Read the model definition and answer for the solid it produces. Units are mm, in the model's axes. Face numbers are marked on the shaded views. A direction names the side the tool comes from. Round coordinates to 2 decimals unless told otherwise and drop trailing zeros. Write each loop counter-clockwise with the first axis right and the second up, starting at its lowest first coordinate (ties: lowest second). Pieces come first, ordered by that corner, then holes. Notation, with made-up numbers: (73, 5.25) -> (131, 5.25) arc R9 cw to (131, 15.25) -> close; hole circle Ø1 at (55, -6.75). An arc over 180 degrees is marked (long way). Return JSON: item names as keys, results as strings. Group by question number.
(1) Straight lines are drawn through the part: line 1 (X direction, y = 6.25, z = 18); line 2 (X direction, y = 6.25, z = 13); line 3 (X direction, y = 3.5, z = 0). For each, find the intervals that lie inside material, in ascending order.
(2) A cutting plane is placed at D-D on z = 0. Give the vertices of the cut face in (x, y), then the cut area to 3 significant figures.
(3) A cutting plane is placed at C-C on y = 1. Give the vertices of the cut face in (x, z).
(4) For the marked faces 4, 5, 6 and 7, determine the directions among +Z, -Z, +X, -X, +Y, -Y from which every point of the face is accessible in a straight line to the end or side of a thin tool.
(5) The mould has two halves that part along X. Classify the marked faces 1, 2 and 3: released by +X, released by -X, zero draft, split by the parting line, or undercut.
(6) A cutting plane is placed at B-B on y = 8.75. Give the vertices of the cut face in (x, z).
(7) Given pin 1 (2 mm diameter, centred on x = -0.5, z = 19.5, fed in from +Y); pin 2 (5 mm diameter, centred on x = 19.5, y = 7, fed in from -Z); pin 3 (5 mm diameter, centred on y = 7, z = 5, fed in from -X), each flat-ended and moving along its own axis, determine where each tip first touches the part or whether it passes through.
(8) A cutting plane is placed at A-A on x = 0. Give the vertices of the cut face in (y, z), then the cut area to 4 significant figures.
```python
from build123d import *

# Parameters (mm, degrees)
SKETCH1_W           = 29.5
SKETCH1_H           = 6.5
SKETCH1_R           = 1.65
SKETCH1_H_2         = 20
BOSS_EXTRUDE1_DEPTH = 5
SKETCH3_W           = 14.6
SKETCH3_H           = 13.25
SKETCH3_W_2         = 14.2
BOSS_EXTRUDE2_DEPTH = 5
SKETCH5_W           = 3
SKETCH5_H           = 13.25
BOSS_EXTRUDE4_DEPTH = 5
BOSS_EXTRUDE5_DEPTH = 2.5


with BuildPart() as part:
    # Sketch1 → Boss-Extrude1 (new body)
    # profile 1 of 2: a face of its own
    with BuildSketch(Plane(origin=(0, 0, 0), x_dir=(1, 0, 0), z_dir=(0, 1, 0))):
        Rectangle(SKETCH1_W, SKETCH1_H)
        with Locations(Location((0, 0, 0), (0, 0, 270))):
            Circle(SKETCH1_R, mode=Mode.SUBTRACT)
    # profile 2 of 2: a face of its own
    with BuildSketch(Plane(origin=(0, 0, 0), x_dir=(1, 0, 0), z_dir=(0, 1, 0))):
        with Locations((0, -13.25)):
            Rectangle(SKETCH1_W, SKETCH1_H_2)
    extrude(amount=BOSS_EXTRUDE1_DEPTH)

    # Sketch3 → Boss-Extrude2 (add)
    with BuildSketch(Plane(origin=(0, 5, 0), x_dir=(1, 0, 0), z_dir=(0, 1, 0))):
        with Locations((22.05, -16.625)):
            Rectangle(SKETCH3_W, SKETCH3_H)
        with Locations((-21.85, -16.625)):
            Rectangle(SKETCH3_W_2, SKETCH3_H)
    extrude(amount=-BOSS_EXTRUDE2_DEPTH)

    # Sketch5 → Boss-Extrude4 (add, symmetric)
    with BuildSketch(Plane(origin=(0, 5, 0), x_dir=(1, 0, 0), z_dir=(0, 1, 0))):
        with Locations((-30.45, -16.625)):
            Rectangle(SKETCH5_W, SKETCH5_H)
        with Locations((30.85, -16.625)):
            Rectangle(SKETCH5_W, SKETCH5_H)
    extrude(amount=BOSS_EXTRUDE4_DEPTH, both=True)

    # Sketch6 → Boss-Extrude5 (add)
    with BuildSketch(Plane(origin=(0, 5, 0), x_dir=(1, 0, 0), z_dir=(0, 1, 0))):
        Polygon((0, -23.25), (7, -23.25), (7, -16.25), (-7, -16.25), (-7, -23.25), align=None)
    extrude(amount=BOSS_EXTRUDE5_DEPTH)


solid = part.part
```
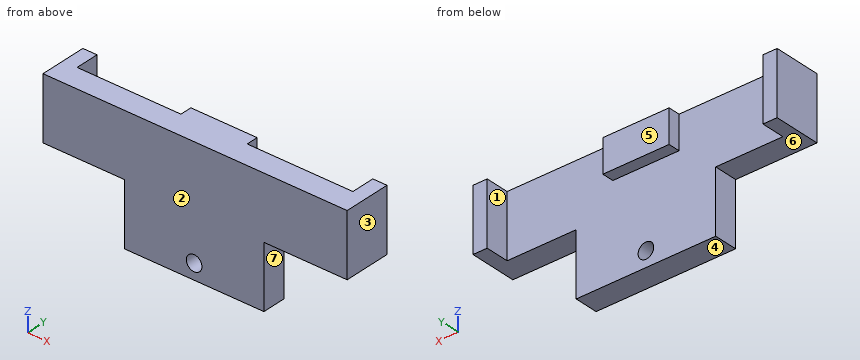
Checks:
{
 "1": {"line 1": "x = -31.95 to -28.95, -7 to 7, 29.35 to 32.35", "line 2": "x = -31.95 to -28.95, 29.35 to 32.35", "line 3": "x = -14.75 to -1.65, 1.65 to 14.75"},
 "2": {"outline": "(-14.75, 0) -> (-1.65, 0) -> (-1.65, 5) -> (-14.75, 5) -> close; (1.65, 0) -> (14.75, 0) -> (14.75, 5) -> (1.65, 5) -> close", "area": "131 mm^2"},
 "3": {"outline": "(-31.95, 10) -> (-14.75, 10) -> (-14.75, -3.25) -> (14.75, -3.25) -> (14.75, 10) -> (32.35, 10) -> (32.35, 23.25) -> (-31.95, 23.25) -> close; hole circle Ø3.3 at (0, 0)"},
 "4": {"face 4": "-Z, +X, -X, +Y, -Y", "face 5": "+Z, -Z, +Y", "face 6": "-Z, -X, +Y, -Y", "face 7": "-Z, +X, +Y, -Y"},
 "5": {"face 1": "undercut", "face 2": "zero draft", "face 3": "released by +X"},
 "6": {"outline": "(-31.95, 10) -> (-28.95, 10) -> (-28.95, 23.25) -> (-31.95, 23.25) -> close; (29.35, 10) -> (32.35, 10) -> (32.35, 23.25) -> (29.35, 23.25) -> close"},
 "7": {"pin 1": "stops at y = 7.5", "pin 2": "stops at z = 10", "pin 3": "stops at x = -14.75"},
 "8": {"outline": "(0, -3.25) -> (5, -3.25) -> (5, -1.65) -> (0, -1.65) -> close; (0, 1.65) -> (5, 1.65) -> (5, 16.25) -> (7.5, 16.25) -> (7.5, 23.25) -> (0, 23.25) -> close", "area": "133.5 mm^2"}
}
